Work out the finished part from the listing and answer in its coordinate system (mm). Face numbers are marked on the shaded views. A direction names the side the tool comes from. Coordinates: 2 decimals unless noted, no trailing zeros. Loops run counter-clockwise (first coordinate to the right, second up) from the corner with the lowest first, then second, coordinate; pieces in that order, holes last. Notation, with made-up numbers: (75.25, 52.25) -> (103.25, 52.25) arc R8 ccw to (103.25, 63.25) -> close; hole circle Ø6 at (7.25, -39.75). An arc over 180 degrees is marked (long way). Use a Markdown table: item, result.
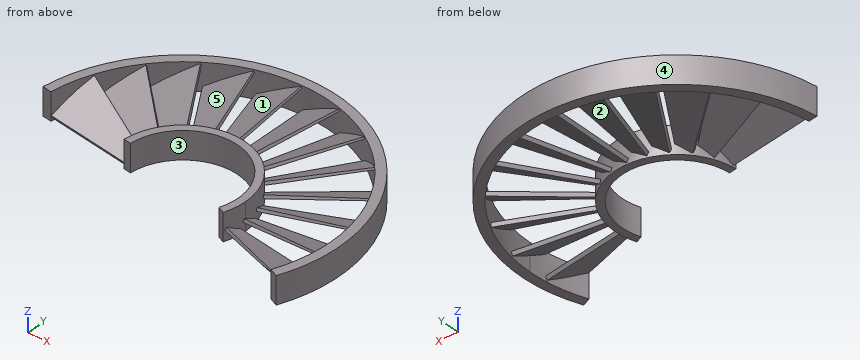
from build123d import *

# Parameters (mm, degrees)
PAD037_DEPTH              = 200
TUBE039_R                 = 100
TUBE039_R_2               = 80
TUBE039_DEPTH             = 200
PAD038_DEPTH              = 100
PAD039_DEPTH              = 2
COMMON018_PLACEMENT_ANGLE = 28
ARRAY016_COUNT            = 22
ARRAY016_PLACEMENT_ANGLE  = 180
TUBE040_R                 = 85
TUBE040_R_2               = 80
TUBE040_DEPTH             = 15
TUBE041_R                 = 34
TUBE041_R_2               = 30
TUBE041_DEPTH             = 15


with BuildPart() as body038:
    # Sketch037 → Pad037 (new body)
    with BuildSketch(Plane.XY):
        Polygon((-29.110853, 1.584928), (-96.197479, 11.61747), (-96.197479, -126.516327), (86.349205, -133.978043), (86.349205, -36.423061), (25.978256, -9.215396), align=None)
    extrude(amount=PAD037_DEPTH)


with BuildPart() as tube039:
    # Tube039 → Tube039 (new body)
    with BuildSketch(Plane.XY):
        Circle(TUBE039_R)
        Circle(TUBE039_R_2, mode=Mode.SUBTRACT)
    extrude(amount=TUBE039_DEPTH)


with BuildPart() as body039:
    # Sketch038 → Pad038 (new body)
    with BuildSketch(Plane.XZ):
        Polygon((0, 0), (0, 2), (26, 0.9), (26, 0), align=None)
    extrude(amount=PAD038_DEPTH)


with BuildPart() as body039_1:
    # Body039 placement: moved
    add(body039.part.moved(Location((-5, 0, 5))))


with BuildPart() as cut012:
    # Sketch039 → Pad039 (new body)
    with BuildSketch(Plane.XY):
        Polygon((0, 0), (0, -52), (25.94305, -47.924315), (8.5, 0), align=None)
    extrude(amount=PAD039_DEPTH)


with BuildPart() as cut012_1:
    # Body040 placement: moved
    add(cut012.part.moved(Location((-5, -33, 5))))

    # Common018: intersect Body039
    add(body039_1.part, mode=Mode.INTERSECT)


with BuildPart() as cut012_2:
    # Common018 placement: moved
    add(cut012_1.part.rotate(Axis((0, 0, 0), (0, 1, 0)), COMMON018_PLACEMENT_ANGLE))

    # Array016: Cut012 ×22 about axis
    array016_axis = Axis((0, 0, 0), (0, 0, 1))


with BuildPart() as cut012_3:
    add(cut012_2.part)
    for i in range(1, ARRAY016_COUNT):
        add(cut012_2.part.rotate(array016_axis, i * 360 / ARRAY016_COUNT))


with BuildPart() as cut012_4:
    # Array016 placement: moved
    add(cut012_3.part.moved(Location((0, 0, 78))).rotate(Axis((0, 0, 78), (0, 1, 0)), ARRAY016_PLACEMENT_ANGLE))

    # Cut012: cut Tube039
    add(tube039.part, mode=Mode.SUBTRACT)


with BuildPart() as tube040:
    # Tube040 → Tube040 (new body)
    with BuildSketch(Plane.XY.offset(68.5)):
        Circle(TUBE040_R)
        Circle(TUBE040_R_2, mode=Mode.SUBTRACT)
    extrude(amount=TUBE040_DEPTH)


with BuildPart() as stator2h2:
    # Tube041 → Tube041 (new body)
    with BuildSketch(Plane.XY.offset(68.5)):
        Circle(TUBE041_R)
        Circle(TUBE041_R_2, mode=Mode.SUBTRACT)
    extrude(amount=TUBE041_DEPTH)

    # Fusion018: union Cut012, Tube040
    add(cut012_4.part)
    add(tube040.part)

    # Cut013: cut Body038
    add(body038.part, mode=Mode.SUBTRACT)


solid = stator2h2.part
Q1. For the marked faces 1, 2 and 3, determine the directions among +Z, -Z, +X, -X, +Y, -Y from which every point of the face is accessible in a straight line to the end or side of a thin tool.
Solved:
| item | result |
|---|---|
| face 1 | +Z |
| face 2 | -Z |
| face 3 | +Z, -Z |
Q2. Given pin 1 Ø1 at (x, z) = (9, 71.5) entering from -Y; pin 2 Ø1.5 at (y, z) = (40, 79.5) entering from +X; pin 3 Ø5 at (x, y) = (66.5, 27.5) entering from +Z, each flat-ended and moving along its own axis, determine where each tip first touches the part or whether it passes through.
Solved:
| item | result |
|---|---|
| pin 1 | y = 28.46 |
| pin 2 | x = 75.4 |
| pin 3 | z = 75.05 |
Q3. Section A-A on y = 71 is taken. Determine the outline of the cut face in (x, z).
Solved:
| item | result |
|---|---|
| outline | (-46.73, 68.5) -> (-36.86, 68.5) -> (-36.86, 74.46) -> (-23.52, 81.06) -> (-24, 82.01) -> (-36.86, 76.26) -> (-36.86, 83.5) -> (-46.73, 83.5) -> close; (-23, 71.24) -> (-22.02, 69.47) -> (-2.63, 80.4) -> (-3.12, 81.38) -> close; (-2.07, 71.24) -> (-1.13, 69.47) -> (18.15, 80.79) -> (17.65, 81.72) -> close; (18.69, 71.24) -> (19.67, 69.47) -> (36.86, 79.16) -> (36.86, 68.5) -> (46.73, 68.5) -> (46.73, 83.5) -> (36.86, 83.5) -> (36.86, 80.51) -> close |
Q4. Consider line 1 (Y direction, x = 0, z = 73); line 2 (X direction, y = 64, z = 78.75). Determine where each line is inside the solid, lowest interval first. Write a range as [from, to].
Solved:
| item | result |
|---|---|
| line 1 | [30, 34], [80, 85] |
| line 2 | [-55.94, -48], [-26.79, -23.69], [-6.22, -3.5], [12.06, 14.67], [31.36, 34.08], [48, 55.94] |
Q5. Section B-B on x = -53.5 is taken. Determine the outline of the cut face in (y, z), and give its area (3 significant figures).
Solved:
| item | result |
|---|---|
| outline | (5.6, 71.24) -> (6.55, 69.47) -> (21.26, 78.02) -> (20.62, 79.14) -> close; (22.16, 71.24) -> (23.19, 69.47) -> (42.81, 79.95) -> (42.13, 80.9) -> close; (43.62, 71.24) -> (44.86, 69.47) -> (59.48, 75.96) -> (59.48, 68.5) -> (66.05, 68.5) -> (66.05, 83.5) -> (59.48, 83.5) -> (59.48, 77.61) -> close |
| area | 192 mm² |
Q6. Section C-C on y = 37.5 is taken. State how many separate pieces and enclosed holes the cut face has, and give its area (3 significant figures).
Solved:
| item | result |
|---|---|
| separate pieces | 8 |
| enclosed holes | 0 |
| area | 405 mm² |
Q7. Determine the mould class of the marked faces 4 and 5 for opening direction X: pulls with the +X half, pulls with the -X half, needs draft (parallel to the pull), parting line crosses it, or undercut.
Solved:
| item | result |
|---|---|
| face 4 | parting line crosses it |
| face 5 | undercut |
